```python
from build123d import *
from build123d.topology import SkipClean

# Parameters (mm, degrees)
BOSS_EXTRUDE1_DEPTH   = 12
BOSS_EXTRUDE1_2_DEPTH = 12
BOSS_EXTRUDE2_DEPTH   = 43.5
SKETCH9_W             = 16.09
SKETCH9_H             = 12.33
BOSS_EXTRUDE3_DEPTH   = 12.5
SKETCH10_W            = 12.33
SKETCH10_H            = 16.09
BOSS_EXTRUDE4_DEPTH   = 12.5
BOSS_EXTRUDE5_START   = 22.85
SKETCH11_W            = 12.33
SKETCH11_H            = 16.09
SKETCH11_W_2          = 16.09
SKETCH11_H_2          = 12.33
BOSS_EXTRUDE5_DEPTH   = 8.15
SKETCH21_W            = 34.892896775
SKETCH21_H            = 3.983406167
SKETCH21_W_2          = 3.397806166
SKETCH21_H_2          = 35.53848689
BOSS_EXTRUDE8_DEPTH   = 12
SKETCH13_W            = 0.82460559
SKETCH13_H            = 22.85
CUT_EXTRUDE1_DEPTH    = 16.09
SKETCH14_W            = 0.915845165
SKETCH14_H            = 22.85
CUT_EXTRUDE2_DEPTH    = 16.09
SKETCH15_W            = 2.3
SKETCH15_H            = 12
BOSS_EXTRUDE6_DEPTH   = 39.09
SKETCH16_W            = 3.5
SKETCH16_H            = 12
BOSS_EXTRUDE7_DEPTH   = 39.09
SKETCH17_W            = 10.950625106
SKETCH17_H            = 21.5
SKETCH17_W_2          = 21.501773634
SKETCH17_H_2          = 11.67953826
CUT_EXTRUDE3_DEPTH    = 31.5
CUT_EXTRUDE4_START    = 65
SKETCH18_R            = 1.825
CUT_EXTRUDE4_DEPTH    = 11
CIRPATTERN1_COUNT     = 8
SKETCH19_R            = 1.5
CUT_EXTRUDE5_DEPTH    = 5
SKETCH20_R            = 1.5
CUT_EXTRUDE8_DEPTH    = 5
SKETCH22_W            = 5
SKETCH22_H            = 12.65
SKETCH22_W_2          = 12.65
SKETCH22_H_2          = 5
CUT_EXTRUDE9_DEPTH    = 12
FILLET1_R             = 7
CUT_EXTRUDE10_DEPTH   = 12
CUT_EXTRUDE11_DEPTH   = 12
SKETCH25_W            = 13.245845165
SKETCH25_H            = 0.617327952
SKETCH25_H_2          = 0.5
CUT_EXTRUDE12_DEPTH   = 16.09
SKETCH26_W            = 13.15460559
SKETCH26_H            = 0.716542238
SKETCH26_H_2          = 0.793164057
CUT_EXTRUDE13_DEPTH   = 16.09


with BuildPart() as part:
    # Sketch8 → Boss-Extrude1 (new body)
    with BuildSketch(Plane(origin=(0, 0, 0), x_dir=(1, 0, 0), z_dir=(0, 1, 0))):
        with BuildLine():
            Line((-39.48619564, -18.776596206), (-17.984422006, -18.776596206))
            Line((-17.984422006, -18.776596206), (-17.984422006, -18.772777241))
            Line((-17.984422006, -18.772777241), (12.857426144, -18.772777241))
            Line((12.857426144, -18.772777241), (20.062824101, -25.857862934))
            Line((20.062824101, -25.857862934), (20.062824101, -16.775))
            Line((20.062824101, -16.775), (25.897828719, -16.775))
            Line((25.897828719, -16.775), (20.099516291, -11.073504999))
            Line((20.099516291, -11.073504999), (20.099516291, 21.123910655))
            Line((20.099516291, 21.123910655), (53.873878262, 21.123910655))
            Line((53.873878262, 21.123910655), (53.873878262, -16.775))
            Line((53.873878262, -16.775), (62.798084167, -16.775))
            ThreePointArc((62.798084167, -16.775), (64.447170112, -8.459448243), (65, 0))
            ThreePointArc((65, 0), (-28.795809447, 58.273504771), (-39.48619564, -51.63177659))
            Line((-39.48619564, -51.63177659), (-39.48619564, -18.776596206))
        make_face()
        Polygon((12.655697004, 12.655697004), (17.288003611, -4.632306606), (4.632306606, -17.288003611), (-12.655697004, -12.655697004), (-17.288003611, 4.632306606), (-4.632306606, 17.288003611), align=None, mode=Mode.SUBTRACT)
    extrude(amount=BOSS_EXTRUDE1_DEPTH)



with BuildPart() as body_2:
    # Sketch8 → Boss-Extrude1 2 (new body)
    with BuildSketch(Plane(origin=(0, 0, 0), x_dir=(1, 0, 0), z_dir=(0, 1, 0))):
        with BuildLine():
            Line((-17.984422006, -55.432543879), (-17.984422006, -62.462473255))
            ThreePointArc((-17.984422006, -62.462473255), (21.088153384, -61.484061242), (52.535934131, -38.275))
            Line((52.535934131, -38.275), (20.062824101, -38.275))
            Line((20.062824101, -38.275), (20.062824101, -25.857862934))
            Line((20.062824101, -25.857862934), (19.864525542, -55.432543879))
            Line((19.864525542, -55.432543879), (-17.984422006, -55.432543879))
        make_face()
    extrude(amount=BOSS_EXTRUDE1_2_DEPTH)


with BuildPart() as part_1:
    add(part.part)

    add(body_2.part)  # Boss-Extrude2 merges body 2
    # Sketch8_4 → Boss-Extrude2 (add)
    with BuildSketch(Plane(origin=(0, 0, 0), x_dir=(1, 0, 0), z_dir=(0, 1, 0))):
        with BuildLine():
            Line((-34.074422006, -38.525), (-17.984422006, -38.525))
            Line((-17.984422006, -38.525), (-17.984422006, -18.776596206))
            Line((-17.984422006, -18.776596206), (-39.48619564, -18.776596206))
            Line((-39.48619564, -18.776596206), (-39.48619564, -51.63177659))
            ThreePointArc((-39.48619564, -51.63177659), (-29.241134908, -58.051322373), (-17.984422006, -62.462473255))
            Line((-17.984422006, -62.462473255), (-17.984422006, -55.432543879))
            Line((-17.984422006, -55.432543879), (-17.984422006, -50.855))
            Line((-17.984422006, -50.855), (-34.074422006, -50.855))
            Line((-34.074422006, -50.855), (-34.074422006, -38.525))
        make_face()
        with BuildLine():
            Line((20.062824101, -16.775), (20.062824101, -25.857862934))
            Line((20.062824101, -25.857862934), (20.062824101, -38.275))
            Line((20.062824101, -38.275), (52.535934131, -38.275))
            ThreePointArc((52.535934131, -38.275), (58.660433379, -27.999170628), (62.798084167, -16.775))
            Line((62.798084167, -16.775), (53.873878262, -16.775))
            Line((53.873878262, -16.775), (50.855, -16.775))
            Line((50.855, -16.775), (50.855, -32.865))
            Line((50.855, -32.865), (38.525, -32.865))
            Line((38.525, -32.865), (38.525, -16.775))
            Line((38.525, -16.775), (25.897828719, -16.775))
            Line((25.897828719, -16.775), (20.062824101, -16.775))
        make_face()
    extrude(amount=BOSS_EXTRUDE2_DEPTH)

    # Sketch9 → Boss-Extrude3 (add)
    with BuildSketch(Plane.XZ):
        with Locations((-26.029422006, 44.69)):
            Rectangle(SKETCH9_W, SKETCH9_H)
    extrude(amount=-BOSS_EXTRUDE3_DEPTH)

    # Sketch10 → Boss-Extrude4 (add)
    with BuildSketch(Plane.XZ):
        with Locations((44.69, 24.82)):
            Rectangle(SKETCH10_W, SKETCH10_H)
    extrude(amount=-BOSS_EXTRUDE4_DEPTH)

    # Sketch11 → Boss-Extrude5 (add)
    with BuildSketch(Plane(origin=(0, 12.5, 0), x_dir=(1, 0, 0), z_dir=(0, 1, 0)).offset(BOSS_EXTRUDE5_START)):
        with Locations((44.69, -24.82)):
            Rectangle(SKETCH11_W, SKETCH11_H)
        with Locations((-26.029422006, -44.69)):
            Rectangle(SKETCH11_W_2, SKETCH11_H_2)
    extrude(amount=BOSS_EXTRUDE5_DEPTH)

    # Sketch21 → Boss-Extrude8 (add)
    with BuildSketch(Plane(origin=(0, 12, 0), x_dir=(1, 0, 0), z_dir=(0, 1, 0))):
        with Locations((-0.537973619, -20.764480324)):
            Rectangle(SKETCH21_W, SKETCH21_H)
        with Locations((21.798419374, 3.35466721)):
            Rectangle(SKETCH21_W_2, SKETCH21_H_2)
    extrude(amount=-BOSS_EXTRUDE8_DEPTH)

    # Sketch13 → Cut-Extrude1 (cut)
    with BuildSketch(Plane(origin=(-17.984422006, 0, 0), x_dir=(0, 0, -1), z_dir=(1, 0, 0))):
        with Locations((-38.112697205, 23.925)):
            Rectangle(SKETCH13_W, SKETCH13_H)
    extrude(amount=-CUT_EXTRUDE1_DEPTH, mode=Mode.SUBTRACT)

    # Sketch14 → Cut-Extrude2 (cut)
    with BuildSketch(Plane(origin=(0, 0, 16.775), x_dir=(-1, 0, 0), z_dir=(0, 0, -1))):
        with Locations((-38.067077418, 23.925)):
            Rectangle(SKETCH14_W, SKETCH14_H)
    extrude(amount=-CUT_EXTRUDE2_DEPTH, mode=Mode.SUBTRACT)

    # Sketch15 → Boss-Extrude6 (add)
    with BuildSketch(Plane(origin=(0, 0, 16.775), x_dir=(-1, 0, 0), z_dir=(0, 0, -1))):
        with Locations((-52.723878262, 6)):
            Rectangle(SKETCH15_W, SKETCH15_H)
    extrude(amount=BOSS_EXTRUDE6_DEPTH)

    # Sketch16 → Boss-Extrude7 (add)
    with BuildSketch(Plane(origin=(-17.984422006, 0, 0), x_dir=(0, 0, -1), z_dir=(1, 0, 0))):
        with Locations((-53.682543879, 6)):
            Rectangle(SKETCH16_W, SKETCH16_H)
    extrude(amount=BOSS_EXTRUDE7_DEPTH)

    # Sketch17 → Cut-Extrude3 (cut)
    with BuildSketch(Plane(origin=(0, 43.5, 0), x_dir=(1, 0, 0), z_dir=(0, 1, 0))):
        with Locations((25.538136654, -27.525)):
            Rectangle(SKETCH17_W, SKETCH17_H)
        with Locations((-28.735308823, -24.616365336)):
            Rectangle(SKETCH17_W_2, SKETCH17_H_2)
    extrude(amount=-CUT_EXTRUDE3_DEPTH, mode=Mode.SUBTRACT)

    # Sketch18 → Cut-Extrude4 (cut)
    with SkipClean():  # the faces are left unmerged after this step: merging them gives an invalid solid
        with BuildSketch(Plane.XY.offset(CUT_EXTRUDE4_START)):
            with Locations((0, 6)):
                Circle(SKETCH18_R)
        cut_extrude4 = extrude(amount=-CUT_EXTRUDE4_DEPTH, mode=Mode.SUBTRACT)

    # CirPattern1: Cut-Extrude4 ×8 about axis
    with SkipClean():  # the faces are left unmerged after this step: merging them gives an invalid solid
        cirpattern1_axis = Axis((0, 0, 0), (0, 1, 0))
        for i in range(1, CIRPATTERN1_COUNT):
            add(cut_extrude4.rotate(cirpattern1_axis, i * 360 / CIRPATTERN1_COUNT), mode=Mode.SUBTRACT)

    # Sketch19 → Cut-Extrude5 (cut)
    with SkipClean():  # the faces are left unmerged after this step: merging them gives an invalid solid
        with BuildSketch(Plane(origin=(0, 0, 16.775), x_dir=(-1, 0, 0), z_dir=(0, 0, -1))):
            with Locations((-44.69, 38.75)):
                Circle(SKETCH19_R)
            with Locations((-44.69, 8.95)):
                Circle(SKETCH19_R)
        extrude(amount=-CUT_EXTRUDE5_DEPTH, mode=Mode.SUBTRACT)

    # Sketch20 → Cut-Extrude8 (cut)
    with SkipClean():  # the faces are left unmerged after this step: merging them gives an invalid solid
        with BuildSketch(Plane(origin=(-17.984422006, 0, 0), x_dir=(0, 0, -1), z_dir=(1, 0, 0))):
            with Locations((-44.69, 38.75)):
                Circle(SKETCH20_R)
            with Locations((-44.69, 8.95)):
                Circle(SKETCH20_R)
        extrude(amount=-CUT_EXTRUDE8_DEPTH, mode=Mode.SUBTRACT)

    # Sketch22 → Cut-Extrude9 (cut)
    with SkipClean():  # the faces are left unmerged after this step: merging them gives an invalid solid
        with BuildSketch(Plane(origin=(0, 43.5, 0), x_dir=(1, 0, 0), z_dir=(0, 1, 0))):
            with Locations((-31.574422006, -44.53)):
                Rectangle(SKETCH22_W, SKETCH22_H)
            with Locations((44.53, -30.365)):
                Rectangle(SKETCH22_W_2, SKETCH22_H_2)
        extrude(amount=-CUT_EXTRUDE9_DEPTH, mode=Mode.SUBTRACT)

    # Fillet1
    fillet1_edges = [part_1.edges().sort_by_distance(p)[0] for p in [
        (-17.984422006, 6, 22.756183408),
        (23.497322457, 6, -21.123910655),
        (51.573878262, 6, -21.123910655),
        (19.88799308, 6, 51.932543879),
    ]]
    fillet(fillet1_edges, radius=FILLET1_R)

    # Sketch23 → Cut-Extrude10 (cut)
    with SkipClean():  # the faces are left unmerged after this step: merging them gives an invalid solid
        with BuildSketch(Plane(origin=(0, 12, 0), x_dir=(1, 0, 0), z_dir=(0, 1, 0))):
            with BuildLine():
                Line((-3.988594308, -22.756183408), (2.962026381, -22.756183408))
                ThreePointArc((2.962026381, -22.756183408), (-0.513283963, -21.31666273), (-3.988594308, -22.756183408))
            make_face()
        extrude(amount=-CUT_EXTRUDE10_DEPTH, mode=Mode.SUBTRACT)

    # Sketch24 → Cut-Extrude11 (cut)
    with SkipClean():  # the faces are left unmerged after this step: merging them gives an invalid solid
        with BuildSketch(Plane(origin=(0, 12, 0), x_dir=(1, 0, 0), z_dir=(0, 1, 0))):
            with BuildLine():
                Line((23.497322457, -3.301623153), (23.497322457, 3.156615754))
                ThreePointArc((23.497322457, 3.156615754), (22.159777385, -0.072503699), (23.497322457, -3.301623153))
            make_face()
        extrude(amount=-CUT_EXTRUDE11_DEPTH, mode=Mode.SUBTRACT)

    # Sketch25 → Cut-Extrude12 (cut)
    with SkipClean():  # the faces are left unmerged after this step: merging them gives an invalid solid
        with BuildSketch(Plane(origin=(0, 0, 16.775), x_dir=(-1, 0, 0), z_dir=(0, 0, -1))):
            with Locations((-44.232077418, 35.658663976)):
                Rectangle(SKETCH25_W, SKETCH25_H)
            with Locations((-44.232077418, 12.25)):
                Rectangle(SKETCH25_W, SKETCH25_H_2)
        extrude(amount=-CUT_EXTRUDE12_DEPTH, mode=Mode.SUBTRACT)

    # Sketch26 → Cut-Extrude13 (cut)
    with SkipClean():  # the faces are left unmerged after this step: merging them gives an invalid solid
        with BuildSketch(Plane(origin=(-17.984422006, 0, 0), x_dir=(0, 0, -1), z_dir=(1, 0, 0))):
            with Locations((-44.277697205, 35.708271119)):
                Rectangle(SKETCH26_W, SKETCH26_H)
            with Locations((-44.277697205, 12.103417972)):
                Rectangle(SKETCH26_W, SKETCH26_H_2)
        extrude(amount=-CUT_EXTRUDE13_DEPTH, mode=Mode.SUBTRACT)


solid = part_1.part
```
For this review, take the finished solid that the model builds, in its own axes (mm). A direction names the side the tool comes from. Coordinates: 2 decimals unless noted, no trailing zeros. Loops run counter-clockwise (first coordinate to the right, second up) from the corner with the lowest first, then second, coordinate; pieces in that order, holes last. Notation, with made-up numbers: (10, 14.25) - (21, 14.25) arc R35 ccw to (21, 47.25) - close; hole circle Ø1 at (9.5, 49.5). An arc over 180 degrees is marked (long way). Use one line per item in the form item = value. Start each with the question number.
1) Draft analysis for pull direction Y (two halves, no side actions). For faces 1 (the face through (-22.984, 9, 45)), 2 (the face through (-15, 12, -15)), 3 (the face through (31.013, 28, 28)), state which applies: released by +Y, released by -Y, zero draft, split by the parting line, or undercut.
2) For faces 4 (the face through (0, 6, 54)), 5 (the face through (59.58, 4.22, 0.4)), 6 (the face through (44, 40, 27.865)), 7 (the face through (-11.05, 5.92, -10.87)), list the 3-axis set-ups (+Z, -Z, +X, -X, +Y, -Y) from which the entire face can be reached by the end or side of a thin tool; tool diameter is ignored.
3) Take a section at B-B (x = 0). State the section outline as (y, z) points (3 decimals), plus the area to 3 significant figures.
4) Take a section at C-C (z = -32). State the section outline as (x, y) points.
5) To check wall thickness, follow probe 1 along Y at (x, z) = (59, 0) (3 decimals); probe 2 along Y at (x, z) = (-20.15, 44.69); probe 3 along X at (y, z) = (37, 44). State the ranges of each line that lie inside material, in increasing order. Write a range as from..to.
6) For pin 1 (5 mm diameter, centred on x = 30.5, y = 30.5, fed in from +Z) (3 decimals); pin 2 (4 mm diameter, centred on x = 44.69, y = 8.95, fed in from +Z); pin 3 (10 mm diameter, centred on y = 17.5, z = 36.5, fed in from +X), all flat-tipped, find the tip position at first contact; note any pin that passes through.
7) Take a section at A-A (y = 30.5). State the section outline as (x, z) points (3 decimals).
From the geometry:
q1.face_1 = undercut
q1.face_2 = released by +Y
q1.face_3 = zero draft
q2.face_4 = +Z
q2.face_5 = +X
q2.face_6 = +Y
q2.face_7 = +Y, -Y
q3.outline = (0, -65) - (4.175, -65) - (4.175, -54) - (7.825, -54) - (7.825, -65) - (12, -65) - (12, -16.047) - (0, -16.047) - close; (0, 16.047) - (12, 16.047) - (12, 21.344) - (0, 21.344) - close; (0, 51.933) - (12, 51.933) - (12, 65) - (7.825, 65) - (7.825, 54) - (4.175, 54) - (4.175, 65) - (0, 65) - close
q3.area = 728 mm2
q4.outline = (-56.58, 0) - (56.58, 0) - (56.58, 12) - (-56.58, 12) - close
q5.probe_1 = 0..4.175, 7.825..12
q5.probe_2 = 0..7.45, 10.45..11.71, 36.07..37.25, 40.25..43.5
q5.probe_3 = -39.49..-34.07, -29.07..-17.98
q6.pin_1 = 38.275
q6.pin_2 = 49.02
q6.pin_3 = 56.86
q7.outline = (-39.486, 30.456) - (-17.984, 30.456) - (-17.984, 37.7) - (-34.074, 37.7) - (-34.074, 50.855) - (-17.984, 50.855) - (-17.984, 62.462) arc R65 ccw to (-39.486, 51.632) - close; (31.013, 16.775) - (37.609, 16.775) - (37.609, 32.865) - (50.855, 32.865) - (50.855, 16.775) - (62.798, 16.775) arc R65 ccw to (52.536, 38.275) - (31.013, 38.275) - close
